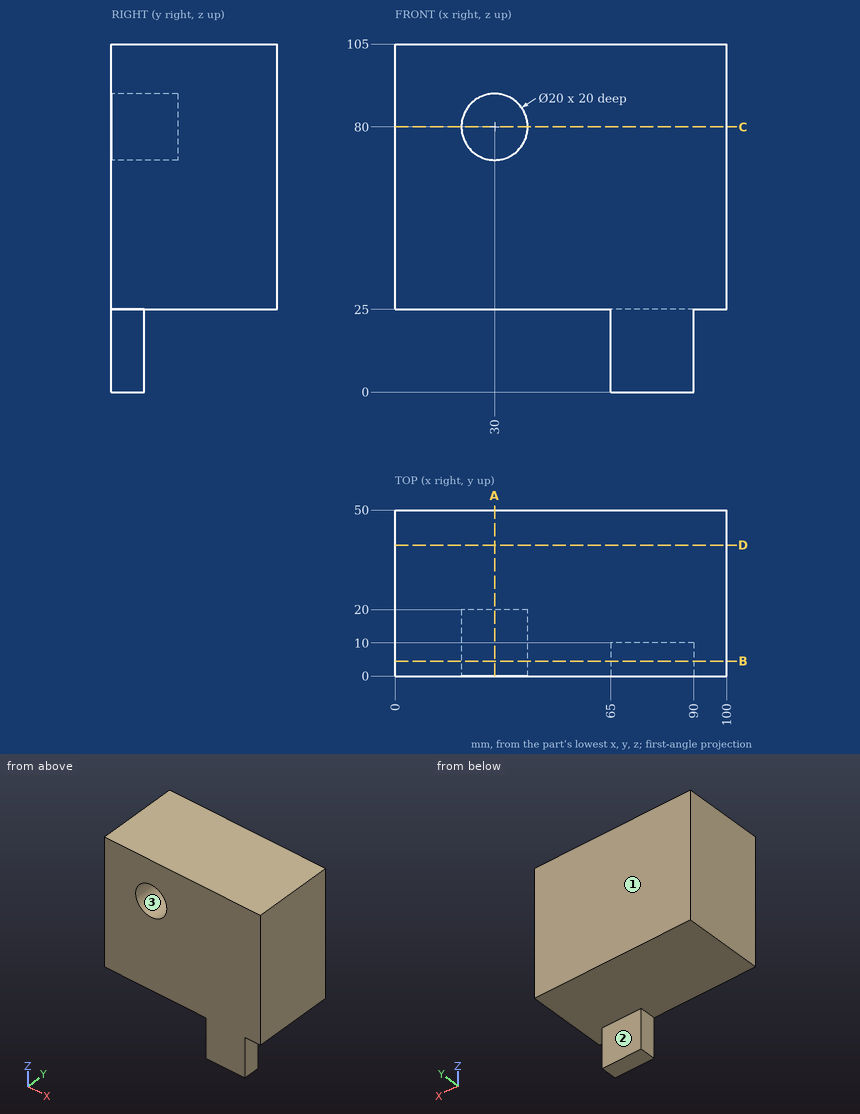
Source: three-view drawing plus pictorial views. Frame: mm from the lowest corner of the part. A direction names the side the tool comes from. Round coordinates to 2 decimals unless told otherwise and drop trailing zeros. Write each loop counter-clockwise with the first axis right and the second up, starting at its lowest first coordinate (ties: lowest second). Pieces come first, ordered by that corner, then holes. Notation, with made-up numbers: M 50.5,53.25 L 109.5,53.25 A23 cw 109.5,82.25 Z; hole C -17,46 d4. An arc over 180 degrees is marked long. Write item = value, one per line.
Item 1: Material intervals for line 1 along Z through (x, y) = (30, 10); line 2 along Y through (x, z) = (27, 77); line 3 along Z through (x, y) = (78, 48), sorted ascending. Write a range as [from, to].
Findings:
line_1 = [25, 70], [90, 105]
line_2 = [20, 50]
line_3 = [25, 105]
Item 2: Section query D-D on y = 39.5. Return loops of the section in (x, z).
Findings:
outline = M 0,25 L 100,25 L 100,105 L 0,105 Z
Item 3: Section query A-A on x = 30. Return loops of the section in (y, z), then the cut area to 3 significant figures.
Findings:
outline = M 0,25 L 50,25 L 50,105 L 0,105 L 0,90 L 20,90 L 20,70 L 0,70 Z
area = 3,600 mm^2
Item 4: Section query C-C on z = 80. Return loops of the section in (x, y), then the cut area to 3 significant figures.
Findings:
outline = M 0,0 L 20,0 L 20,20 L 40,20 L 40,0 L 100,0 L 100,50 L 0,50 Z
area = 4,600 mm^2
Item 5: Access query for the marked faces 1, 2 and 3. Directions: +Z, -Z, +X, -X, +Y, -Y. A direction counts if a zero-diameter tool reaches every point of the face in a straight line with its end or side. Return the directions, or none.
Findings:
face_1 = +Z, -Z, +X, -X, +Y
face_2 = -Z, +X, -X, +Y
face_3 = -Y
Item 6: Section query B-B on y = 4.5. Return loops of the section in (x, z), then the cut area to 3 significant figures.
Findings:
outline = M 0,25 L 65,25 L 65,0 L 90,0 L 90,25 L 100,25 L 100,105 L 0,105 Z; hole C 30,80 d20
area = 8,310 mm^2
Item 7: Pin query (flat end, axial travel): P1, Ø6, axis at x = 33.5, z = 77.5, coming from the -Y side; P2, Ø2, axis at x = 15.5, y = 28, coming from the -Z side; P3, Ø8, axis at y = 3.5, z = 13, coming from the -X side. Return the tip coordinate at first contact, or that it passes through.
Findings:
P1 = 20
P2 = 25
P3 = 65
